Part print with two shaded views. Sizes in mm from the minimum x, y, z corner. A direction names the side the tool comes from. Coordinates: 2 decimals unless noted, no trailing zeros. Order: outer loops, then holes, each group sorted by start corner. A loop starts at its lowest first (then second) coordinate and runs counter-clockwise, first axis right, second up. Notation, with made-up numbers: (-26, 40.5) - (-16, 40.5) arc R26 ccw to (-16, 57.5) - close; hole circle Ø4 at (-16.5, -37.75). An arc over 180 degrees is marked (long way). Write each question's results on one line, items separated by ' | '. Start each with the question number.
Q1. Wall check: probe 1 along X at (y, z) = (3.75, 7); probe 2 along X at (y, z) = (6.75, 11.25); probe 3 along Y at (x, z) = (24, 6.25). Give the ranges that are in metal, low to high.
Q2. Pin check, flat tips, straight feed: P1, Ø3, axis at y = 5.5, z = 6.5, coming from the -X side; P2, Ø4, axis at x = 24.5, y = 6, coming from the -Z side; P3, Ø2, axis at x = 26, z = 3.5, coming from the -Y side. Stop position of each tip, or through.
Q3. Band-saw the part on D-D, the plane z = 11.5. Write the cut outline in (x, y).
Q4. Band-saw the part on B-B, the plane z = 6.5. Write the cut outline in (x, y).
Q5. Pull direction Y, two halves, no side cores. Call the marked faces 1, 2 and 3: released by +Y, released by -Y, zero draft, split by the parting line, or undercut.
Q6. Which spindle directions (+Z, -Z, +X, -X, +Y, -Y) get a long thin tool onto all of the face, cutting with end or side? Do the marked faces 4, 5 and 6. Say none if no direction does.
Q7. Band-saw the part on C-C, the plane x = 13.5. Write the cut outline in (y, z), then the cut area to 3 significant figures.
Q8. Band-saw the part on A-A, the plane x = 2.5. Write the cut outline in (y, z), then the cut area to 3 significant figures.
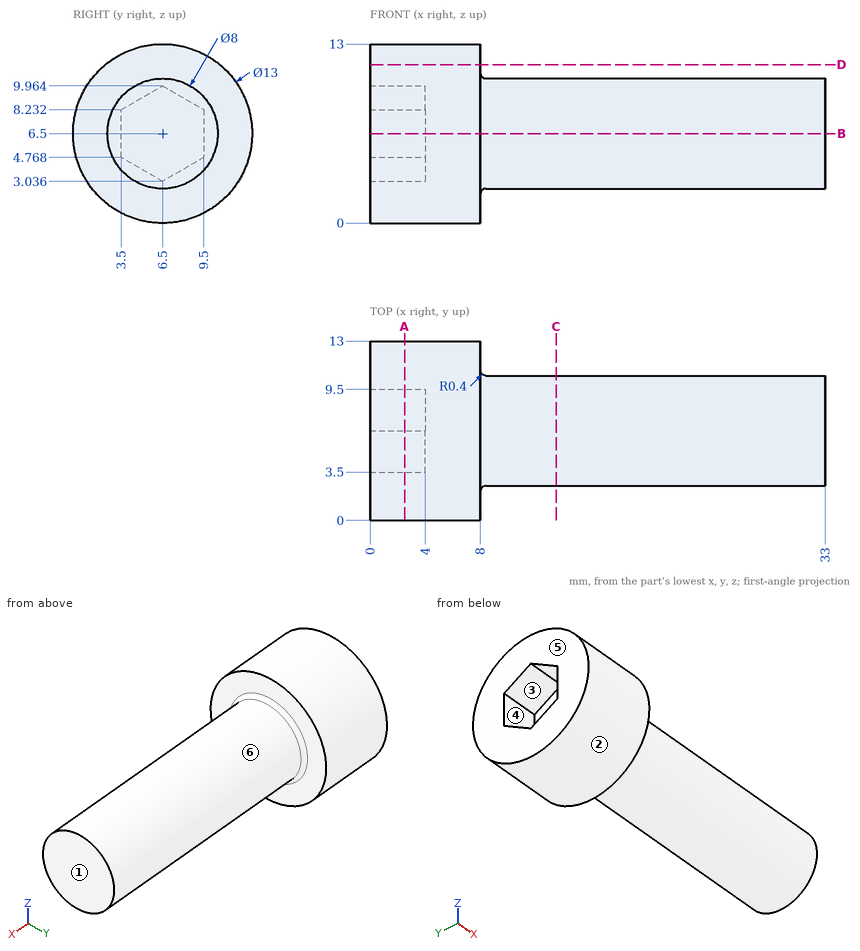
Results below:
1) probe 1: x = 4 to 33 | probe 2: x = 0 to 8 | probe 3: y = 2.51 to 10.49
2) P1: stops at x = 4 | P2: stops at z = 2.5 | P3: stops at y = 3.04
3) outline: (0, 2.35) - (8, 2.35) - (8, 10.65) - (0, 10.65) - close
4) outline: (0, 0) - (8, 0) - (8, 2.1) arc R0.4 cw to (8.4, 2.5) - (33, 2.5) - (33, 10.5) - (8.4, 10.5) arc R0.4 cw to (8, 10.9) - (8, 13) - (0, 13) - (0, 9.5) - (4, 9.5) - (4, 3.5) - (0, 3.5) - close
5) face 1: zero draft | face 2: split by the parting line | face 3: undercut
6) face 4: -X | face 5: +Z, -Z, -X, +Y, -Y | face 6: +X
7) outline: circle Ø8 at (6.5, 6.5) | area: 50.3 mm²
8) outline: circle Ø13 at (6.5, 6.5); hole (3.5, 4.77) - (6.5, 3.04) - (9.5, 4.77) - (9.5, 8.23) - (6.5, 9.96) - (3.5, 8.23) - close | area: 102 mm²
